from build123d import *

# Parameters (mm, degrees)
SKETCH_1_W      = 40
SKETCH_1_H      = 30
SKETCH_1_R      = 1.5
EXTRUDE_1_DEPTH = 3
FILLET_1_R      = 5


with BuildPart() as part:
    # 草圖1 → 填料-伸長1 (new body)
    with BuildSketch(Plane.XY):
        Rectangle(SKETCH_1_W, SKETCH_1_H)
        with Locations((-12, 7)):
            Circle(SKETCH_1_R, mode=Mode.SUBTRACT)
        with Locations((-12, -7)):
            Circle(SKETCH_1_R, mode=Mode.SUBTRACT)
        with Locations(Location((12, -7, 0), (0, 0, 180))):
            Circle(SKETCH_1_R, mode=Mode.SUBTRACT)
        with Locations(Location((12, 7, 0), (0, 0, 180))):
            Circle(SKETCH_1_R, mode=Mode.SUBTRACT)
    extrude(amount=EXTRUDE_1_DEPTH)

    # 圓角1
    fillet_1_edges = [part.edges().sort_by_distance(p)[0] for p in [
        (-20, 15, 1.5),
        (20, 15, 1.5),
    ]]
    fillet(fillet_1_edges, radius=FILLET_1_R)


solid = part.part
CAD build for the part. Positions are in the model's coordinates, mm. Give positions to 0.01 mm unless a question says otherwise; leave off trailing zeros. Loops run counter-clockwise (first coordinate to the right, second up) from the corner with the lowest first, then second, coordinate; pieces in that order, holes last. Notation, with made-up numbers: M 1,11.25 L 36,11.25 A8 cw 36,26.25 Z; hole C 31.25,-31.5 d11. An arc over 180 degrees is marked long. Answer in a Markdown table with one row per item. Add a question column.
Item 1: Band-saw the part on C-C on z = 2.3. Give the cut face in (x, y).
Item 2: Band-saw the part on B-B on y = 7. Give the cut face in (x, z).
Item 3: Band-saw the part on A-A on x = -12. Give the cut face in (y, z).
Item 4: Probe probe 1 along Y at (x, z) = (-12, 1.8); probe 2 along Y at (x, z) = (-12.5, 1.4); probe 3 along X at (y, z) = (-8.25, 0.45). List the from-to ranges inside material, lowest first.
Item 5: Drop a flat-ended pin along its axis: P1, Ø2.5, axis at x = 12, y = 7, coming from the -Z side. Give the stop position or say it passes through.
Item 6: Mould opens along Y. For faces 1 (the face through (0, 0, 3)), 2 (the face through (13.2, 7.9, 1.5)), 3 (the face through (-19, 13, 2)) say: +Y half, -Y half, draft (parallel to the pull), parting line (faces both ways), or undercut.
Reply:
| question | item | result |
|---|---|---|
| 1 | outline | M -20,-15 L 20,-15 L 20,10 A5 ccw 15,15 L -15,15 A5 ccw -20,10 Z; hole C -12,-7 d3; hole C -12,7 d3; hole C 12,-7 d3; hole C 12,7 d3 |
| 2 | outline | M -20,0 L -13.5,0 L -13.5,3 L -20,3 Z; M -10.5,0 L 10.5,0 L 10.5,3 L -10.5,3 Z; M 13.5,0 L 20,0 L 20,3 L 13.5,3 Z |
| 3 | outline | M -15,0 L -8.5,0 L -8.5,3 L -15,3 Z; M -5.5,0 L 5.5,0 L 5.5,3 L -5.5,3 Z; M 8.5,0 L 15,0 L 15,3 L 8.5,3 Z |
| 4 | probe 1 | y = -15 to -8.5, -5.5 to 5.5, 8.5 to 15 |
| 4 | probe 2 | y = -15 to -8.41, -5.59 to 5.59, 8.41 to 15 |
| 4 | probe 3 | x = -20 to -12.83, -11.17 to 11.17, 12.83 to 20 |
| 5 | P1 | passes through |
| 6 | face 1 | draft |
| 6 | face 2 | undercut |
| 6 | face 3 | +Y half |
